Read the model definition and answer for the solid it produces. Units are mm, in the model's axes. A direction names the side the tool comes from. Give positions to 0.01 mm unless a question says otherwise; leave off trailing zeros. Order: outer loops, then holes, each group sorted by start corner. A loop starts at its lowest first (then second) coordinate and runs counter-clockwise, first axis right, second up. Notation, with made-up numbers: (-31.5, -32.5) - (12.5, -32.5) arc R18 cw to (12.5, -23.5) - close; hole circle Ø4 at (-9.5, 1.25). An arc over 180 degrees is marked (long way). Write each question's results on one line, items separated by ' | '.
from build123d import *

# Parameters (mm, degrees)
SKETCH1_W           = 57.999999262
SKETCH1_H           = 28.000000864
BOSS_EXTRUDE1_DEPTH = 8
CUT_EXTRUDE10_REACH = 59.565
SKETCH11_R          = 1.6
CUT_EXTRUDE11_DEPTH = 58.565336436
CUT_EXTRUDE12_DEPTH = 58.565336436
SKETCH15_W          = 5.000000121
SKETCH15_H          = 4.999999888
BOSS_EXTRUDE2_DEPTH = 4.999998957
SKETCH16_W          = 4.999998957
SKETCH16_H          = 4.999999888
BOSS_EXTRUDE3_DEPTH = 4.999998957
BOSS_EXTRUDE4_DEPTH = 85
HOLE2_START         = -8.343500085
HOLE2_OUTLINE_R     = 5
HOLE2_DEPTH         = 57.999999262
FILLET1_R           = 5


# Read off the part's stored shape, not the designer's step: Hole2
with BuildPart() as part:
    # Sketch1 → Boss-Extrude1 (new body)
    with BuildSketch(Plane.XZ):
        with Locations((20.656499546, 14.000000432)):
            Rectangle(SKETCH1_W, SKETCH1_H)
    extrude(amount=BOSS_EXTRUDE1_DEPTH)

    # Sketch11 → Cut-Extrude10 (cut, up to next)
    with BuildSketch(Plane.XZ.offset(8), mode=Mode.PRIVATE) as cut_extrude10_sk1:
        with Locations(Location((20.656499132, 2.749998098, 0), (0, 0, 270))):
            Circle(SKETCH11_R)
    cut_extrude10_tool1 = extrude(cut_extrude10_sk1.sketch, amount=-CUT_EXTRUDE10_REACH, mode=Mode.PRIVATE) & part.part
    add(cut_extrude10_tool1.solids().sort_by_distance((20.656499, -8, 2.749998))[0], mode=Mode.SUBTRACT)

    # Sketch12 → Cut-Extrude11 (cut, through all)
    with BuildSketch(Plane(origin=(0, -8, 0), x_dir=(-1, 0, 0), z_dir=(0, 1, 0))):
        Polygon((-7.388492115, 18.547229469), (-7.506358903, 18.799999729), (-7.666328922, 19.028460607), (-7.863540202, 19.225670025), (-8.092000149, 19.385639578), (-8.344767615, 19.503509626), (-8.614162914, 19.575690851), (-8.891999722, 19.600000232), (-9.16983746, 19.575690851), (-9.439231828, 19.503509626), (-9.692000225, 19.385639578), (-9.920460172, 19.225670025), (-10.11766959, 19.028460607), (-10.277640074, 18.799999729), (-10.395510122, 18.547229469), (-10.467690416, 18.277840689), (-10.491999798, 17.999999225), (-10.467690416, 17.722159624), (-10.395510122, 17.452770844), (-10.277640074, 17.200000584), (-10.11766959, 16.971539706), (-9.920460172, 16.774330288), (-9.692000225, 16.614360735), (-9.439231828, 16.496490687), (-9.16983746, 16.424309462), (-8.891999722, 16.40000008), (-8.614162914, 16.424309462), (-8.344767615, 16.496490687), (-8.092000149, 16.614360735), (-7.863540202, 16.774330288), (-7.666328922, 16.971539706), (-7.506358903, 17.200000584), (-7.388492115, 17.452770844), (-7.316308096, 17.722159624), (-7.292000111, 17.999999225), (-7.316308096, 18.277840689), align=None)
    extrude(amount=CUT_EXTRUDE11_DEPTH, mode=Mode.SUBTRACT)

    # Sketch13 → Cut-Extrude12 (cut, through all)
    with BuildSketch(Plane.XZ.offset(8)):
        Polygon((32.698839903, 16.424309462), (32.968230546, 16.496490687), (33.220998943, 16.614360735), (33.449459821, 16.774330288), (33.646669239, 16.971539706), (33.806640655, 17.200000584), (33.92450884, 17.452770844), (33.996690065, 17.722159624), (34.021001309, 17.999999225), (33.996690065, 18.277840689), (33.92450884, 18.547229469), (33.806640655, 18.799999729), (33.646669239, 19.028460607), (33.449459821, 19.225670025), (33.220998943, 19.385639578), (32.968230546, 19.503509626), (32.698839903, 19.575690851), (32.421000302, 19.600000232), (32.143160701, 19.575690851), (31.873770058, 19.503509626), (31.621001661, 19.385639578), (31.392540783, 19.225670025), (31.195329502, 19.028460607), (31.035359949, 18.799999729), (30.917489901, 18.547229469), (30.845310539, 18.277840689), (30.820999295, 17.999999225), (30.845310539, 17.722159624), (30.917489901, 17.452770844), (31.035359949, 17.200000584), (31.195329502, 16.971539706), (31.392540783, 16.774330288), (31.621001661, 16.614360735), (31.873770058, 16.496490687), (32.143160701, 16.424309462), (32.421000302, 16.40000008), align=None)
    extrude(amount=-CUT_EXTRUDE12_DEPTH, mode=Mode.SUBTRACT)

    # Sketch15 → Boss-Extrude2 (add)
    with BuildSketch(Plane.XZ.offset(8)):
        with Locations((-5.843500025, 2.499999944)):
            Rectangle(SKETCH15_W, SKETCH15_H)
    extrude(amount=BOSS_EXTRUDE2_DEPTH)

    # Sketch16 → Boss-Extrude3 (add)
    with BuildSketch(Plane.XZ.offset(8)):
        with Locations((47.156499698, 2.499999944)):
            Rectangle(SKETCH16_W, SKETCH16_H)
    extrude(amount=BOSS_EXTRUDE3_DEPTH)

    # Sketch17 → Boss-Extrude4 (add)
    with BuildSketch(Plane(origin=(0, 0, 0), x_dir=(1, 0, 0), z_dir=(0, 1, 0))):
        Polygon((-8.343500085, 0), (49.656499177, 0), (49.656499177, -8), (49.656499177, -28.000000864), (40.656499177, -28.000000864), (40.656499177, -8), (0.656499915, -8), (0.656499915, -28.000000864), (-8.343500085, -28.000000864), (-8.343500085, -8), align=None)
    extrude(amount=BOSS_EXTRUDE4_DEPTH)

    # Hole2 outline → Hole2 (cut)
    with BuildSketch(Plane.YZ.offset(HOLE2_START)):
        with Locations((73.288734932, 16.920895282)):
            Circle(HOLE2_OUTLINE_R)
    extrude(amount=HOLE2_DEPTH, mode=Mode.SUBTRACT)

    # Fillet1
    fillet1_edges = [part.edges().sort_by_distance(p)[0] for p in [
        (20.656499546, 0, 8),
    ]]
    fillet(fillet1_edges, radius=FILLET1_R)


solid = part.part
(1) Section C-C (x = 18) is taken. Give the vertices of the cut face in (y, z), plus the area to 3 significant figures.
Conclusion:
outline: (-8, 0) - (85, 0) - (85, 8) - (5, 8) arc R5 cw to (0, 13) - (0, 28) - (-8, 28) - close | area: 909 mm^2
(2) Consider probe 1 along X at (y, z) = (58, 17.5); probe 2 along Z at (x, y) = (37, 63); probe 3 along Y at (x, z) = (3, 3.75). Determine where each line is inside the solid, lowest interval first. Write a range as [from, to].
Conclusion:
probe 1: [-8.34, 0.66], [40.66, 49.66] | probe 2: [0, 8] | probe 3: [-8, 85]
(3) For faces 4 (the face through (0.656, 42, 18)), 5 (the face through (44.657, -10, 2)), 6 (the face through (19.683, -4.056, 4.02)), 7 (the face through (47, -10, 5)), determine the directions among +Z, -Z, +X, -X, +Y, -Y from which every point of the face is accessible in a straight line to the end or side of a thin tool.
Conclusion:
face 4: +Z, +Y | face 5: +Z, -Z, -Y | face 6: -Y | face 7: +Z, +X, -X, -Y
(4) Each of these flat-tipped pins is pushed along its axis until it touches: pin 1 (8 mm diameter, centred on x = 40, z = 11.5, fed in from -Y); pin 2 (1.5 mm diameter, centred on x = -5, y = -10.5, fed in from +Z); pin 3 (5 mm diameter, centred on x = 5.5, z = 25, fed in from +Y). Where does it stop, or does it pass through?
Conclusion:
pin 1: y = -8 | pin 2: z = 5 | pin 3: y = 0
(5) The mould has two halves that part along Y. Classify faces 1 (the face through (-3.907, 68.294, 17.141)), 2 (the face through (42, 31, 28)), 3 (the face through (-6, -13, 3)): pulls with the +Y half, pulls with the -Y half, needs draft (parallel to the pull), parting line crosses it, or undercut.
Conclusion:
face 1: undercut | face 2: needs draft | face 3: pulls with the -Y half
(6) Section A-A (y = 2) is taken. Give the vertices of the cut face in (x, z), plus the area to 3 significant figures.
Conclusion:
outline: (-8.34, 0) - (49.66, 0) - (49.66, 28) - (40.66, 28) - (40.66, 9) - (0.66, 9) - (0.66, 28) - (-8.34, 28) - close | area: 864 mm^2
(7) Section D-D (z = 9.5) is taken. Give the vertices of the cut face in (x, y).
Conclusion:
outline: (-8.34, -8) - (49.66, -8) - (49.66, 85) - (40.66, 85) - (40.66, 1.43) - (0.66, 1.43) - (0.66, 85) - (-8.34, 85) - close
(8) Section B-B (z = 14.25) is taken. Give the vertices of the cut face in (x, y), plus the area to 3 significant figures.
Conclusion:
outline: (-8.34, -8) - (49.66, -8) - (49.66, 69.06) - (40.66, 69.06) - (40.66, 0) - (0.66, 0) - (0.66, 69.06) - (-8.34, 69.06) - close; (-8.34, 77.52) - (0.66, 77.52) - (0.66, 85) - (-8.34, 85) - close; (40.66, 77.52) - (49.66, 77.52) - (49.66, 85) - (40.66, 85) - close | area: 1,840 mm^2
